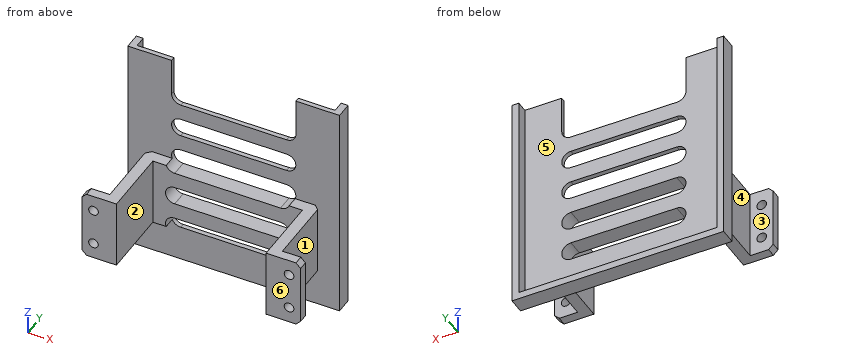
from build123d import *

# Parameters (mm, degrees)
BOSS_EXTRUDE1_DEPTH      = 30
SKETCH2_W                = 50
SKETCH2_H                = 20
CUT_EXTRUDE1_DEPTH       = 30
CHAMFER1_SIZE            = 2
SKETCH3_R                = 2.1
CUT_EXTRUDE2_DEPTH       = 30
SKETCH6_W                = 5
SKETCH6_H                = 30
BOSS_EXTRUDE2_DEPTH      = 5
SKETCH8_W                = 50
SKETCH8_H                = 20
BOSS_EXTRUDE3_DEPTH      = 5
SKETCH9_W                = 25
SKETCH9_H                = 30
BOSS_EXTRUDE4_DEPTH      = 5
SKETCH10_W               = 25
SKETCH10_H               = 30
BOSS_EXTRUDE5_DEPTH      = 5
SKETCH12_W               = 10
SKETCH12_H               = 30
CUT_EXTRUDE3_DEPTH       = 10
SKETCH13_R               = 2.1
CUT_EXTRUDE4_DEPTH       = 10
CHAMFER2_SIZE            = 2
SKETCH14_W               = 6.64500098
SKETCH14_H               = 11.940236137
SKETCH14_W_2             = 7.060313542
SKETCH14_H_2             = 8.410079366
BOSS_EXTRUDE6_DEPTH      = 5
SKETCH15_R               = 2.1
CUT_EXTRUDE5_DEPTH       = 5
SKETCH17_W               = 86
SKETCH17_H               = 93
SKETCH17_W_2             = 71
SKETCH17_H_2             = 30
BOSS_EXTRUDE7_DEPTH      = 2
BOSS_EXTRUDE8_DEPTH      = 5
BOSS_EXTRUDE8_DEPTH_BACK = 2
CUT_EXTRUDE7_DEPTH       = 18
CUT_EXTRUDE8_DEPTH       = 1
SKETCH22_W               = 54
SKETCH22_H               = 16.5
CUT_EXTRUDE9_DEPTH       = 10


with BuildPart() as part:
    # Sketch1 → Boss-Extrude1 (new body)
    with BuildSketch(Plane.XY):
        Polygon((-57.5, -17.5), (-37.5, -17.5), (-32.5, -17.5), (-32.5, 12.5), (32.5, 12.5), (32.5, -17.5), (37.5, -17.5), (57.5, -17.5), (57.5, -12.5), (37.5, -12.5), (37.5, 17.5), (-37.5, 17.5), (-37.5, -12.5), (-57.5, -12.5), align=None)
    extrude(amount=BOSS_EXTRUDE1_DEPTH)

    # Sketch2 → Cut-Extrude1 (cut)
    with BuildSketch(Plane(origin=(0, 17.5, 0), x_dir=(1, 0, 0), z_dir=(0, 1, 0))):
        with Locations((0, -15)):
            Rectangle(SKETCH2_W, SKETCH2_H)
    extrude(amount=-CUT_EXTRUDE1_DEPTH, mode=Mode.SUBTRACT)

    # Chamfer1
    chamfer1_edges = [part.edges().sort_by_distance(p)[0] for p in [
        (-37.5, 17.5, 15),
        (37.5, 17.5, 15),
    ]]
    chamfer(chamfer1_edges, length=CHAMFER1_SIZE)

    # Sketch3 → Cut-Extrude2 (cut)
    with BuildSketch(Plane(origin=(0, -12.5, 0), x_dir=(1, 0, 0), z_dir=(0, 1, 0))):
        with Locations((-47.5, -15)):
            Circle(SKETCH3_R)
        with Locations((47.5, -15)):
            Circle(SKETCH3_R)
    extrude(amount=-CUT_EXTRUDE2_DEPTH, mode=Mode.SUBTRACT)

    # Sketch6 → Boss-Extrude2 (add)
    with BuildSketch(Plane(origin=(0, 17.5, 0), x_dir=(1, 0, 0), z_dir=(0, 1, 0))):
        with Locations((0, -15)):
            Rectangle(SKETCH6_W, SKETCH6_H)
    extrude(amount=-BOSS_EXTRUDE2_DEPTH)

    # Sketch8 → Boss-Extrude3 (add)
    with BuildSketch(Plane(origin=(0, 17.5, 0), x_dir=(1, 0, 0), z_dir=(0, 1, 0))):
        with Locations((0, -15)):
            Rectangle(SKETCH8_W, SKETCH8_H)
    extrude(amount=-BOSS_EXTRUDE3_DEPTH)

    # Sketch9 → Boss-Extrude4 (add)
    with BuildSketch(Plane(origin=(0, -17.5, 0), x_dir=(-1, 0, 0), z_dir=(0, -1, 0))):
        with Locations((45, -15)):
            Rectangle(SKETCH9_W, SKETCH9_H)
    extrude(amount=-BOSS_EXTRUDE4_DEPTH)

    # Sketch10 → Boss-Extrude5 (add)
    with BuildSketch(Plane(origin=(0, -17.5, 0), x_dir=(-1, 0, 0), z_dir=(0, -1, 0))):
        with Locations((-45, -15)):
            Rectangle(SKETCH10_W, SKETCH10_H)
    extrude(amount=-BOSS_EXTRUDE5_DEPTH)

    # Sketch12 → Cut-Extrude3 (cut)
    with BuildSketch(Plane(origin=(0, -12.5, 0), x_dir=(1, 0, 0), z_dir=(0, 1, 0))):
        with Locations((52.5, -15)):
            Rectangle(SKETCH12_W, SKETCH12_H)
        with Locations((-52.5, -15)):
            Rectangle(SKETCH12_W, SKETCH12_H)
    extrude(amount=-CUT_EXTRUDE3_DEPTH, mode=Mode.SUBTRACT)

    # Sketch13 → Cut-Extrude4 (cut)
    with BuildSketch(Plane(origin=(0, -12.5, 0), x_dir=(1, 0, 0), z_dir=(0, 1, 0))):
        with Locations((-42.5, -15)):
            Circle(SKETCH13_R)
        with Locations((42.5, -15)):
            Circle(SKETCH13_R)
    extrude(amount=-CUT_EXTRUDE4_DEPTH, mode=Mode.SUBTRACT)

    # Chamfer2
    chamfer2_edges = [part.edges().sort_by_distance(p)[0] for p in [
        (47.5, -15, 0),
        (-47.5, -15, 0),
        (-47.5, -15, 30),
        (47.5, -15, 30),
    ]]
    chamfer(chamfer2_edges, length=CHAMFER2_SIZE)

    # Sketch14 → Boss-Extrude6 (add)
    with BuildSketch(Plane(origin=(0, -12.5, 0), x_dir=(1, 0, 0), z_dir=(0, 1, 0))):
        with Locations((42.569537531, -14.480859299)):
            Rectangle(SKETCH14_W, SKETCH14_H)
        with Locations((-42.25805311, -15)):
            Rectangle(SKETCH14_W_2, SKETCH14_H_2)
    extrude(amount=-BOSS_EXTRUDE6_DEPTH)

    # Sketch15 → Cut-Extrude5 (cut)
    with BuildSketch(Plane(origin=(0, -12.5, 0), x_dir=(1, 0, 0), z_dir=(0, 1, 0))):
        with Locations((-42.5, -7)):
            Circle(SKETCH15_R)
        with Locations((-42.5, -23)):
            Circle(SKETCH15_R)
        with Locations((42.5, -23)):
            Circle(SKETCH15_R)
        with Locations((42.5, -7)):
            Circle(SKETCH15_R)
    extrude(amount=-CUT_EXTRUDE5_DEPTH, mode=Mode.SUBTRACT)

    # Sketch17 → Boss-Extrude7 (add)
    with BuildSketch(Plane(origin=(0, 17.5, 0), x_dir=(1, 0, 0), z_dir=(0, 1, 0))):
        with Locations((0, -31.5)):
            Rectangle(SKETCH17_W, SKETCH17_H)
        with Locations((0, -15)):
            Rectangle(SKETCH17_W_2, SKETCH17_H_2, mode=Mode.SUBTRACT)
        with Locations((0, -15)):
            Rectangle(SKETCH17_W_2, SKETCH17_H_2)
    extrude(amount=BOSS_EXTRUDE7_DEPTH)

    # Sketch18 → Boss-Extrude8 (add, two sides)
    with BuildSketch(Plane(origin=(0, 19.5, 0), x_dir=(1, 0, 0), z_dir=(0, 1, 0))) as boss_extrude8_sk:
        Polygon((-46, 18), (-46, -78), (-43, -78), (-43, 15), (43, 15), (43, -78), (46, -78), (46, 18), align=None)
    extrude(amount=BOSS_EXTRUDE8_DEPTH)
    extrude(boss_extrude8_sk.sketch, amount=-BOSS_EXTRUDE8_DEPTH_BACK)

    # Sketch19 → Cut-Extrude7 (cut)
    with BuildSketch(Plane(origin=(0, 19.5, 0), x_dir=(1, 0, 0), z_dir=(0, 1, 0))):
        with BuildLine():
            Line((-23, 2.5), (23, 2.5))
            ThreePointArc((23, 2.5), (27, -1.5), (23, -5.5))
            Line((23, -5.5), (-23, -5.5))
            ThreePointArc((-23, -5.5), (-27, -1.5), (-23, 2.5))
        make_face()
        with BuildLine():
            Line((-23, -12.5), (23, -12.5))
            ThreePointArc((23, -12.5), (27, -16.5), (23, -20.5))
            Line((23, -20.5), (-23, -20.5))
            ThreePointArc((-23, -20.5), (-27, -16.5), (-23, -12.5))
        make_face()
        with BuildLine():
            Line((-23, -27.5), (23, -27.5))
            ThreePointArc((23, -27.5), (27, -31.5), (23, -35.5))
            Line((23, -35.5), (-23, -35.5))
            ThreePointArc((-23, -35.5), (-27, -31.5), (-23, -27.5))
        make_face()
        with BuildLine():
            Line((-23, -50.5), (23, -50.5))
            ThreePointArc((23, -50.5), (27, -46.5), (23, -42.5))
            Line((23, -42.5), (-23, -42.5))
            ThreePointArc((-23, -42.5), (-27, -46.5), (-23, -50.5))
        make_face()
        with BuildLine():
            Line((-23, -65.5), (23, -65.5))
            ThreePointArc((23, -65.5), (27, -61.5), (23, -57.5))
            Line((23, -57.5), (-23, -57.5))
            ThreePointArc((-23, -57.5), (-27, -61.5), (-23, -65.5))
        make_face()
    extrude(amount=-CUT_EXTRUDE7_DEPTH, mode=Mode.SUBTRACT)

    # Sketch21 → Cut-Extrude8 (cut)
    with BuildSketch(Plane(origin=(0, -12.5, 0), x_dir=(1, 0, 0), z_dir=(0, 1, 0))):
        Polygon((-37.5, 0), (-37.5, -30), (-45.5, -30), (-47.5, -28), (-47.5, -2), (-45.5, 0), align=None)
        Polygon((37.5, 0), (37.5, -30), (45.5, -30), (47.5, -28), (47.5, -2), (45.5, 0), align=None)
    extrude(amount=-CUT_EXTRUDE8_DEPTH, mode=Mode.SUBTRACT)

    # Sketch22 → Cut-Extrude9 (cut)
    with BuildSketch(Plane(origin=(0, 19.5, 0), x_dir=(1, 0, 0), z_dir=(0, 1, 0))):
        with Locations((0, -69.75)):
            Rectangle(SKETCH22_W, SKETCH22_H)
    extrude(amount=-CUT_EXTRUDE9_DEPTH, mode=Mode.SUBTRACT)


solid = part.part
Source: CAD feature listing. Evaluate the final solid. Frame: model axes, mm. Face numbers are marked on the shaded views. A direction names the side the tool comes from. Coordinates: 2 decimals unless noted, no trailing zeros. Loops run counter-clockwise (first coordinate to the right, second up) from the corner with the lowest first, then second, coordinate; pieces in that order, holes last. Notation, with made-up numbers: (26, -7.5) -> (82, -7.5) arc R18 cw to (82, 24.5) -> close; hole circle Ø1 at (-12, 66). An arc over 180 degrees is marked (long way). Answer in a Markdown table with one row per item. Add a question column.
Q1. Ray query, line 1 along X through (y, z) = (-16, 7); line 2 along Z through (x, y) = (-42.5, -15.35); line 3 along X through (y, z) = (-2.5, 5). Return the intervals inside material, ascending.
Q2. Contact query for flat-ended pins moving along their axis: pin 1 Ø24 at (y, z) = (1, 9) entering from +X; pin 2 Ø10 at (x, z) = (-23.5, 0) entering from +Y; pin 3 Ø1 at (y, z) = (18, 72) entering from +X. Output: stop coordinate, or through.
Q3. Pull-direction query (X, two-part tool) for the marked faces 4, 5 and 6; classes: pulls with the +X half, pulls with the -X half, needs draft (parallel to the pull), parting line crosses it, or undercut.
Q4. Section C-C on y = -8.5. Return the cut outline in (x, z), and give its area (3 significant figures).
Q5. Section A-A on x = -12. Return the cut outline in (y, z).
Q6. Section D-D on x = -30. Return the cut outline in (y, z), and give its area (3 significant figures).
Q7. Reachability of the marked faces 1, 2 and 3 from +Z, -Z, +X, -X, +Y, -Y: full face, straight path, thin tool, end or side. Return the list, or none.
Q8. Section B-B on z = 23. Give the number of separate pieces and of enclosed holes in the cut face, and give its area (3 significant figures).
Computed values:
| question | item | result |
|---|---|---|
| 1 | line 1 | x = -47.5 to -44.6, -40.4 to -32.5, 32.5 to 40.4, 44.6 to 47.5 |
| 1 | line 2 | z = 0 to 4.9, 9.1 to 20.9, 25.1 to 30 |
| 1 | line 3 | x = -37.5 to -32.5, 32.5 to 37.5 |
| 2 | pin 1 | stops at x = 37.5 |
| 2 | pin 2 | stops at y = 19.5 |
| 2 | pin 3 | stops at x = 46 |
| 3 | face 4 | pulls with the -X half |
| 3 | face 5 | undercut |
| 3 | face 6 | needs draft |
| 4 | outline | (-37.5, 0) -> (-32.5, 0) -> (-32.5, 30) -> (-37.5, 30) -> close; (32.5, 0) -> (37.5, 0) -> (37.5, 30) -> (32.5, 30) -> close |
| 4 | area | 300 mm^2 |
| 5 | outline | (12.5, 5.5) -> (19.5, 5.5) -> (19.5, 12.5) -> (12.5, 12.5) -> close; (12.5, 20.5) -> (19.5, 20.5) -> (19.5, 27.5) -> (12.5, 27.5) -> close; (17.5, -18) -> (24.5, -18) -> (24.5, -15) -> (19.5, -15) -> (19.5, -2.5) -> (17.5, -2.5) -> close; (17.5, 35.5) -> (19.5, 35.5) -> (19.5, 42.5) -> (17.5, 42.5) -> close; (17.5, 50.5) -> (19.5, 50.5) -> (19.5, 57.5) -> (17.5, 57.5) -> close |
| 6 | outline | (12.5, 0) -> (17.5, 0) -> (17.5, -18) -> (24.5, -18) -> (24.5, -15) -> (19.5, -15) -> (19.5, 78) -> (17.5, 78) -> (17.5, 30) -> (12.5, 30) -> close |
| 6 | area | 357 mm^2 |
| 7 | face 1 | +Z, -Z, +X |
| 7 | face 2 | +Z, -Z, -Y |
| 7 | face 3 | +Z, -Z, -X |
| 8 | separate pieces | 3 |
| 8 | enclosed holes | 0 |
| 8 | area | 931 mm^2 |
